Autodesk Inventor part; units mm, degrees
ref_plane "YZ Plane" through (0, 0, 0) normal (1, 0, 0) x (0, 1, 0)
ref_plane "XZ Plane" through (0, 0, 0) normal (0, 1, 0) x (-1, 0, 0)
ref_plane "XY Plane" through (0, 0, 0) normal (0, 0, 1) x (1, 0, 0)
sketch "Szkic1" plane through (0, 0, 0) normal (0, 1, 0) x (-1, 0, 0)
  line L0 (110, 110) -> (-110, 110)
  line L1 (-110, 110) -> (-110, -110)
  line L2 (-110, -110) -> (110, -110)
  line L3 (110, -110) -> (110, 110)
  line L4 (110, 0) -> (-110, 0) construction
  line L5 (0, 110) -> (0, -110) construction
  point P0 (0, 0)
  dimension "d0" = 220
  dimension "d1" = 220
extrude "Wyciągnięcie proste1" add sketch "Szkic1" along normal blind 3
sketch "Szkic2" plane through (0, 3, 0) normal (0, 1, 0) x (1, 0, 0)
  line L0 (-110, 110) -> (-110, -110)
  line L1 (-110, -110) -> (110, -110)
  line L2 (110, -110) -> (110, 110)
  line L3 (110, 110) -> (-110, 110)
  point P0 (0, 0)
  point P1 (-105, -105)
  point P2 (-105, 105)
  point P3 (105, 105)
  point P4 (105, -105)
  dimension "d4" = 5
  dimension "d5" = 5
  dimension "d6" = 5
  dimension "d7" = 5
hole "Otwór1" at (-105, 3, 105) at (-105, 3, -105) at (105, 3, -105) at (105, 3, 105) direction (0, -1, 0) diameter 3 end through all
fillet "Zaokrąglenie1" radius 3 4 edges at (-110, 1.5, 110) (110, 1.5, 110) (110, 1.5, -110) (-110, 1.5, -110)
chamfer "Faza1" distance 2 angle 45 4 edges at (105, 3, -106.5) (-105, 3, -106.5) (105, 3, 103.5) (-105, 3, 103.5)
properties part number "20_stół"
Geometry check sheet. Reference: the model listing, model coordinates, mm. Coordinates: 2 decimals unless noted, no trailing zeros. Use a Markdown table: item, result. Add a question column.
1. Material ranges on L1, parallel to X at y = 0.35, z = -105, recorded low to high.
2. Go/stop test with a flat-tipped pin: pin 1 Ø4 at (x, z) = (105, -105) entering from +Y. Record where the tip stops, or that it passes through.
3. Mould release check, pull along Z, two halves, no side actions. Record for faces 1 (the face through (106.1, 1.13, -106.2)), 2 (the face through (2, 3, 2)): pulls with the +Z half, pulls with the -Z half, needs draft (parallel to the pull), parting line crosses it, or undercut.
Filled sheet:
| question | item | result |
|---|---|---|
| 1 | L1 | -110 to -106.5, -103.5 to 103.5, 106.5 to 110 |
| 2 | pin 1 | y = 1.5 |
| 3 | face 1 | undercut |
| 3 | face 2 | needs draft |
